Build history of the part. All positions in model axes, mm. Face numbers are marked on the shaded views. A direction names the side the tool comes from. Give positions to 0.01 mm unless a question says otherwise; leave off trailing zeros. Order: outer loops, then holes, each group sorted by start corner. A loop starts at its lowest first (then second) coordinate and runs counter-clockwise, first axis right, second up. Notation, with made-up numbers: M 61,-32.5 L 111,-32.5 A14 cw 111,-6.5 Z; hole C 2.25,-34 d1. An arc over 180 degrees is marked long. Answer as CSV lines item,"result".
from build123d import *

# Parameters (mm, degrees)
SKETCH_R          = 15.5
SKETCH_R_2        = 1.6
PAD_DEPTH         = 3
PAD_FACE5_W       = 19
PAD_FACE5_H       = 3
PAD001_DEPTH      = 12
SKETCH001_W       = 8
SKETCH001_H       = 18.6
PAD002_DEPTH      = 13
PAD002_DEPTH_BACK = 3
PAD003_DEPTH      = 3
PAD004_DEPTH      = 8
SKETCH003_R       = 1.6
POCKET_DEPTH      = 16.001
SKETCH004_R       = 3.2
POCKET001_DEPTH   = 13
SKETCH005_R       = 3.2
POCKET002_DEPTH   = 9
SKETCH006_R       = 1.6
POCKET003_DEPTH   = 21.001


with BuildPart() as part:
    # Sketch → Pad (new body)
    with BuildSketch(Plane.XY):
        with BuildLine():
            Line((-25, 26.5), (-25, 7.5))
            Line((-25, 7.5), (-24.269322, 7.5))
            ThreePointArc((-24.269322, 7.5), (-24.300327, -4.373169), (-18.850224, -14.921604))
            Line((-20.997316, -17.351209), (-18.850224, -14.921604))
            ThreePointArc((-20.997316, -17.351209), (-20.648791, -22.997316), (-15.002684, -22.648791))
            Line((-15.002684, -22.648791), (-12.694657, -20.037077))
            ThreePointArc((-12.694657, -20.037077), (18.733227, -15.054945), (19.812278, 16.747086))
            Line((22.997316, 20.351209), (19.812278, 16.747086))
            ThreePointArc((22.997316, 20.351209), (22.648791, 25.997316), (17.002684, 25.648791))
            Line((17.002684, 25.648791), (13.978579, 22.226778))
            ThreePointArc((13.978579, 22.226778), (7.308575, 25.407838), (0, 26.5))
            Line((-25, 26.5), (0, 26.5))
        make_face()
        Circle(SKETCH_R, mode=Mode.SUBTRACT)
        with Locations((-18, -20)):
            Circle(SKETCH_R_2, mode=Mode.SUBTRACT)
        with Locations((20, 23)):
            Circle(SKETCH_R_2, mode=Mode.SUBTRACT)
    extrude(amount=PAD_DEPTH)

    # Pad Face5 → Pad001 (add)
    with BuildSketch(Plane(origin=(-25, 17, 1.5), x_dir=(0, 1, 0), z_dir=(-1, 0, 0))):
        Rectangle(PAD_FACE5_W, PAD_FACE5_H)
    extrude(amount=PAD001_DEPTH)

    # Sketch001 (on Face15 of Pad001) → Pad002 (join, two sides)
    with BuildSketch(Plane.XY.offset(3)) as pad002_sk:
        with Locations((14.4, 17.2)):
            Rectangle(SKETCH001_W, SKETCH001_H)
    extrude(amount=PAD002_DEPTH)
    extrude(pad002_sk.sketch, amount=-PAD002_DEPTH_BACK)

    # Pad002 Face17 → Pad003 (add)
    with BuildSketch(Plane(origin=(14.369541, 26.5, 8.05167), x_dir=(1, 0, 0), z_dir=(0, 1, 0))):
        Polygon((3.693968, 8.05167), (-3.969541, 8.05167), (-3.969541, -7.94833), (4.030459, -7.94833), (4.030459, 5.05167), (3.693968, 5.05167), align=None)
    extrude(amount=PAD003_DEPTH)

    # Sketch002 (on Face20 of Pad003) → Pad004 (join)
    with BuildSketch(Plane.YZ.offset(18.4)):
        Polygon((7.9, 16), (5.013249, 21), (8.013249, 21), (10.9, 16), align=None)
        Polygon((26.5, 16), (29.5, 16), (32.386751, 21), (29.386751, 21), align=None)
    extrude(amount=-PAD004_DEPTH)

    # Sketch003 (on Face26 of Pad004) → Pocket (cut, through all)
    with BuildSketch(Plane.XY.offset(16)):
        with Locations((14.4, 18.7)):
            Circle(SKETCH003_R)
    extrude(amount=-POCKET_DEPTH, mode=Mode.SUBTRACT)

    # Sketch004 (on Face28 of Pocket) → Pocket001 (cut)
    with BuildSketch(Plane.XY.offset(16)):
        with Locations((20, 23)):
            Circle(SKETCH004_R)
    extrude(amount=-POCKET001_DEPTH, mode=Mode.SUBTRACT)

    # Sketch005 (on Face26 of Pocket001) → Pocket002 (cut)
    with BuildSketch(Plane(origin=(0, 0, 0), x_dir=(1, 0, 0), z_dir=(0, 0, -1))):
        with Locations((14.4, -18.7)):
            Circle(SKETCH005_R)
    extrude(amount=-POCKET002_DEPTH, mode=Mode.SUBTRACT)

    # Sketch006 (on Face2 of Pocket002) → Pocket003 (cut, through all)
    with BuildSketch(Plane(origin=(0, 0, 0), x_dir=(1, 0, 0), z_dir=(0, 0, -1))):
        with Locations((-32.5, -17)):
            Circle(SKETCH006_R)
    extrude(amount=-POCKET003_DEPTH, mode=Mode.SUBTRACT)


solid = part.part
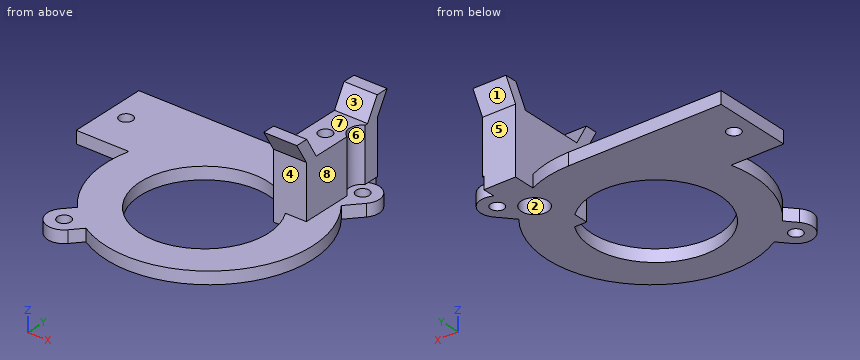
Item 1: Band-saw the part on D-D (x = -32.5). Give the cut face in (y, z).
Geometry says:
outline,"M 7.5,0 L 15.4,0 L 15.4,3 L 7.5,3 Z; M 18.6,0 L 26.5,0 L 26.5,3 L 18.6,3 Z"
Item 2: Band-saw the part on A-A (x = -18). Give the cut face in (y, z).
Geometry says:
outline,"M -24,0 L -21.6,0 L -21.6,3 L -24,3 Z; M -18.4,0 L 26.5,0 L 26.5,3 L -18.4,3 Z"
Item 3: Band-saw the part on B-B (y = 23). Give the cut face in (x, z).
Geometry says:
outline,"M -37,0 L 18.4,0 L 18.4,3 L 16.8,3 L 16.8,16 L 10.4,16 L 10.4,3 L -37,3 Z; M 21.6,0 L 24,0 L 24,3 L 21.6,3 Z"
Item 4: Drop flat-ended pins along their axis: pin 1 (12 mm diameter, centred on y = 14.5, z = 8, fed in from +X); pin 2 (6.5 mm diameter, centred on x = 15.5, z = 8, fed in from -Y); pin 3 (0.9 mm diameter, centred on x = -21.5, z = 1.5, fed in from +Y); pin 4 (10 mm diameter, centred on y = -18.5, z = 9, fed in from +X). Give the stop position or say it passes through.
Geometry says:
pin 1,"stops at x = 23.05"
pin 2,"stops at y = 7.9"
pin 3,"stops at y = 26.5"
pin 4,"passes through"
Item 5: Pull direction Z, two halves, no side cores. Call the marked faces 1, 2, 3 and 4: released by +Z, released by -Z, zero draft, split by the parting line, or undercut.
Geometry says:
face 1,"released by -Z"
face 2,"zero draft"
face 3,"released by +Z"
face 4,"undercut"
Item 6: 3-axis set-ups, long thin cutter, end or side, ignore diameter. For the marked faces 5, 6, 7 and 8: which of +Z, -Z, +X, -X, +Y, -Y reach the whole face in a straight line?
Geometry says:
face 5,"-Z, +X, -X, +Y"
face 6,"+Z, +X"
face 7,"+Z, +X, -X"
face 8,"+Z, +X, +Y, -Y"
Item 7: Band-saw the part on C-C (z = 11.5). Give the cut face in (x, y), and give its area (3 significant figures).
Geometry says:
outline,"M 10.4,7.9 L 18.4,7.9 L 18.4,20.23 A3.2 cw 18.4,25.77 L 18.4,29.5 L 10.4,29.5 Z; hole C 14.4,18.7 d3.2"
area,"158 mm2"
Item 8: Probe line 1 along Y through (x, z) = (14.4, 12.5); line 2 along Z through (x, y) = (-13.5, 14); line 3 along X through (y, z) = (17, 1.05). List the from-to ranges inside material, lowest first. Write a range as from..to.
Geometry says:
line 1,"y = 7.9..17.1, 20.3..29.5"
line 2,"z = 0..3"
line 3,"x = -37..-34.1, -30.9..11.69, 17.11..20.04"
